Work out the finished part from the listing and answer in its coordinate system (mm). A direction names the side the tool comes from. Give positions to 0.01 mm unless a question says otherwise; leave off trailing zeros. Write each loop counter-clockwise with the first axis right and the second up, starting at its lowest first coordinate (ties: lowest second). Pieces come first, ordered by that corner, then holes. Notation, with made-up numbers: (4.5, 31.25) - (12.5, 31.25) arc R22 cw to (12.5, 44.25) - close; hole circle Ø3 at (3, 76.5). An arc over 180 degrees is marked (long way). Write item = value, one per line.
from build123d import *

# Parameters (mm, degrees)
F0_R     = 22.225
F1_DEPTH = 12.7
F0_R_2   = 9.525
F0_R_3   = 14.2875
F2_DEPTH = 22.225


with BuildPart() as f1:
    # F0 (on Front) → F1 (new body, symmetric)
    with BuildSketch(Plane.XZ):
        with BuildLine():
            Line((-35.76122, -1.70331), (-61.16122, -1.70331))
            Line((-61.16122, -1.70331), (22.611454, -23.883373))
            ThreePointArc((22.611454, -23.883373), (41.377511, -19.011414), (54.653603, -4.881791))
            ThreePointArc((54.653603, -4.881791), (62.325841, 3.542555), (73.665641, 4.656909))
            ThreePointArc((73.665641, 4.656909), (92.100975, 1.676194), (102.323325, 17.304685))
            ThreePointArc((102.323325, 17.304685), (97.751671, 43.254331), (84.58042, 66.075425))
            ThreePointArc((84.58042, 66.075425), (70.994806, 72.238394), (57.723636, 65.424647))
            ThreePointArc((57.723636, 65.424647), (42.224433, 55.833223), (27.924188, 67.134716))
            ThreePointArc((27.924188, 67.134716), (28.011866, 66.039385), (28.041119, 64.940939))
            ThreePointArc((28.041119, 64.940939), (5.862071, 44.361094), (-13.003585, 68.015422))
            ThreePointArc((-13.003585, 68.015422), (-28.409448, 45.607643), (-53.983655, 36.365939))
            Line((-53.983655, 36.365939), (-36.843181, 36.365939))
            ThreePointArc((-36.843181, 36.365939), (-17.80087, 17.857139), (-35.76122, -1.70331))
        make_face()
        with Locations((26.453619, 17.315939)):
            Circle(F0_R, mode=Mode.SUBTRACT)
        with BuildLine():
            ThreePointArc((96.303526, 17.315939), (85.178419, 6.236313), (74.053312, 17.315939))
            ThreePointArc((74.053312, 17.315939), (71.1827, 33.595993), (62.9171, 47.912432))
            ThreePointArc((62.9171, 47.912432), (64.258991, 63.620822), (79.961752, 62.214594))
            ThreePointArc((79.961752, 62.214594), (92.091061, 41.206014), (96.303526, 17.315939))
        make_face(mode=Mode.SUBTRACT)
    extrude(amount=F1_DEPTH, both=True)

    # F0 (on Front) → F2 (join, symmetric)
    with BuildSketch(Plane.XZ):
        with BuildLine():
            ThreePointArc((27.312843, 70.375018), (6.197833, 85.543184), (-13.003585, 68.015422))
            ThreePointArc((-13.003585, 68.015422), (5.862071, 44.361094), (28.041119, 64.940939))
            ThreePointArc((28.041119, 64.940939), (28.011866, 66.039385), (27.924188, 67.134716))
            ThreePointArc((27.924188, 67.134716), (27.534155, 68.738951), (27.312843, 70.375018))
        make_face()
        with Locations((7.403619, 64.940939)):
            Circle(F0_R_2, mode=Mode.SUBTRACT)
        with BuildLine():
            ThreePointArc((-62.243181, 36.365939), (-81.285492, 16.77474), (-61.16122, -1.70331))
            Line((-61.16122, -1.70331), (-35.76122, -1.70331))
            ThreePointArc((-35.76122, -1.70331), (-17.80087, 17.857139), (-36.843181, 36.365939))
            Line((-36.843181, 36.365939), (-53.983655, 36.365939))
            ThreePointArc((-53.983655, 36.365939), (-55.579185, 36.337294), (-57.174716, 36.365939))
            Line((-57.174716, 36.365939), (-62.243181, 36.365939))
        make_face()
        with BuildLine():
            Line((-36.843181, 6.216139), (-62.243181, 6.216139))
            ThreePointArc((-62.243181, 6.216139), (-73.342981, 17.315939), (-62.243181, 28.415739))
            Line((-62.243181, 28.415739), (-36.843181, 28.415739))
            ThreePointArc((-36.843181, 28.415739), (-25.743381, 17.315939), (-36.843181, 6.216139))
        make_face(mode=Mode.SUBTRACT)
        with Locations((26.453619, 17.315939)):
            Circle(F0_R)
        with Locations((26.453619, 17.315939)):
            Circle(F0_R_3, mode=Mode.SUBTRACT)
    extrude(amount=F2_DEPTH, both=True)


solid = f1.part
1. For a pull along Z with two mould halves and no side action, classify faces 5 (the cylindrical face through (-73.34, 0.31, 17.07)), 6 (the flat face through (-60, 0, 36.366)), 7 (the flat face through (-19.86, -0.18, -12.64)) as pulls with the +Z half, pulls with the -Z half, needs draft (parallel to the pull), parting line crosses it, or undercut.
Solution:
face_5 = undercut
face_6 = pulls with the +Z half
face_7 = pulls with the -Z half
2. Find section D-D, the plane z = 59. Give the vertices of the cut face in (x, y) (1 decimal), then the cut area to 3 significant figures.
Solution:
outline = (-16.8, -12.7) - (-12.4, -12.7) - (-12.4, -22.2) - (0, -22.2) - (0, 22.2) - (-12.4, 22.2) - (-12.4, 12.7) - (-16.8, 12.7) - close; (14.8, -22.2) - (27.2, -22.2) - (27.2, -12.7) - (33.6, -12.7) - (33.6, 12.7) - (27.2, 12.7) - (27.2, 22.2) - (14.8, 22.2) - close; (52.7, -12.7) - (61, -12.7) - (61, 12.7) - (52.7, 12.7) - close; (82.5, -12.7) - (89.8, -12.7) - (89.8, 12.7) - (82.5, 12.7) - close
area = 1,770 mm^2
3. Straight lines are drawn through the part: line 1 (X direction, y = -5, z = 70); line 2 (X direction, y = -11.5, z = 13); line 3 (X direction, y = -5, z = 21). For each, find the intervals that lie inside material, in ascending order.
Solution:
line_1 = -12.6 to -0.67, 15.47 to 27.35, 62.93 to 79.89
line_2 = -80.8 to -72.47, -26.62 to 12.83, 40.07 to 74.94, 95.41 to 101.76
line_3 = -80.93 to -72.71, -26.37 to 12.65, 40.26 to 73.91, 96.21 to 102.23
4. Find section A-A, the plane y = 16. Give the number of separate pieces and of enclosed holes in the cut face, then the cut area to 3 significant figures.
Solution:
separate_pieces = 3
enclosed_holes = 3
area = 3,120 mm^2
5. Find section B-B, the plane z = 13.5. Give the vertices of the cut face in (x, y) (3 decimals).
Solution:
outline = (-80.907, -22.225) - (-72.666, -22.225) - (-72.666, 22.225) - (-80.907, 22.225) - close; (-26.42, -22.225) - (-18.179, -22.225) - (-18.179, -12.7) - (4.559, -12.7) - (4.559, -22.225) - (12.685, -22.225) - (12.685, 22.225) - (4.559, 22.225) - (4.559, 12.7) - (-18.179, 12.7) - (-18.179, 22.225) - (-26.42, 22.225) - close; (40.222, -22.225) - (48.349, -22.225) - (48.349, -12.7) - (74.745, -12.7) - (74.745, 12.7) - (48.349, 12.7) - (48.349, 22.225) - (40.222, 22.225) - close; (95.612, -12.7) - (101.883, -12.7) - (101.883, 12.7) - (95.612, 12.7) - close
6. A tool of negligible diameter and unlimited length cuts with its end or side. For faces 1 (the cylindrical face through (91.974, -0.178, 41.526)), 2 (the cylindrical face through (23.56, -17.53, 39.35)), 3 (the cylindrical face through (-17.794, 17.529, 17.446)), 4 (the flat face through (-45, -17, 36.366)), from which of +Z, -Z, +X, -X, +Y, -Y can it reach the whole face along a straight path? Write none if from no direction.
Solution:
face_1 = +Y, -Y
face_2 = -Y
face_3 = +Y
face_4 = +Z, -X, -Y
7. Given pin 1 (1.5 mm diameter, centred on y = 7, z = 28, fed in from -X); pin 2 (2 mm diameter, centred on x = 50.5, y = -2, fed in from +Z); pin 3 (2 mm diameter, centred on x = 14.5, y = 12, fed in from -Z); pin 4 (11.5 mm diameter, centred on x = 7.4, z = 64.94, fed in from -Y), each flat-ended and moving along its own axis, determine where each tip first touches the part or whether it passes through.
Solution:
pin_1 = -78.5
pin_2 = 58.19
pin_3 = -22
pin_4 = through
